The drawing under review shows one solid part. Ordinate dimensions are in mm from its lowest x, y, z. A direction names the side the tool comes from. Round coordinates to 2 decimals unless told otherwise and drop trailing zeros. Order: outer loops, then holes, each group sorted by start corner. A loop starts at its lowest first (then second) coordinate and runs counter-clockwise, first axis right, second up. Notation, with made-up numbers: M 61,80.25 L 85,80.25 A32 cw 85,115.25 Z; hole C -2,-28.5 d2. An arc over 180 degrees is marked long. Use a Markdown table: item, result.
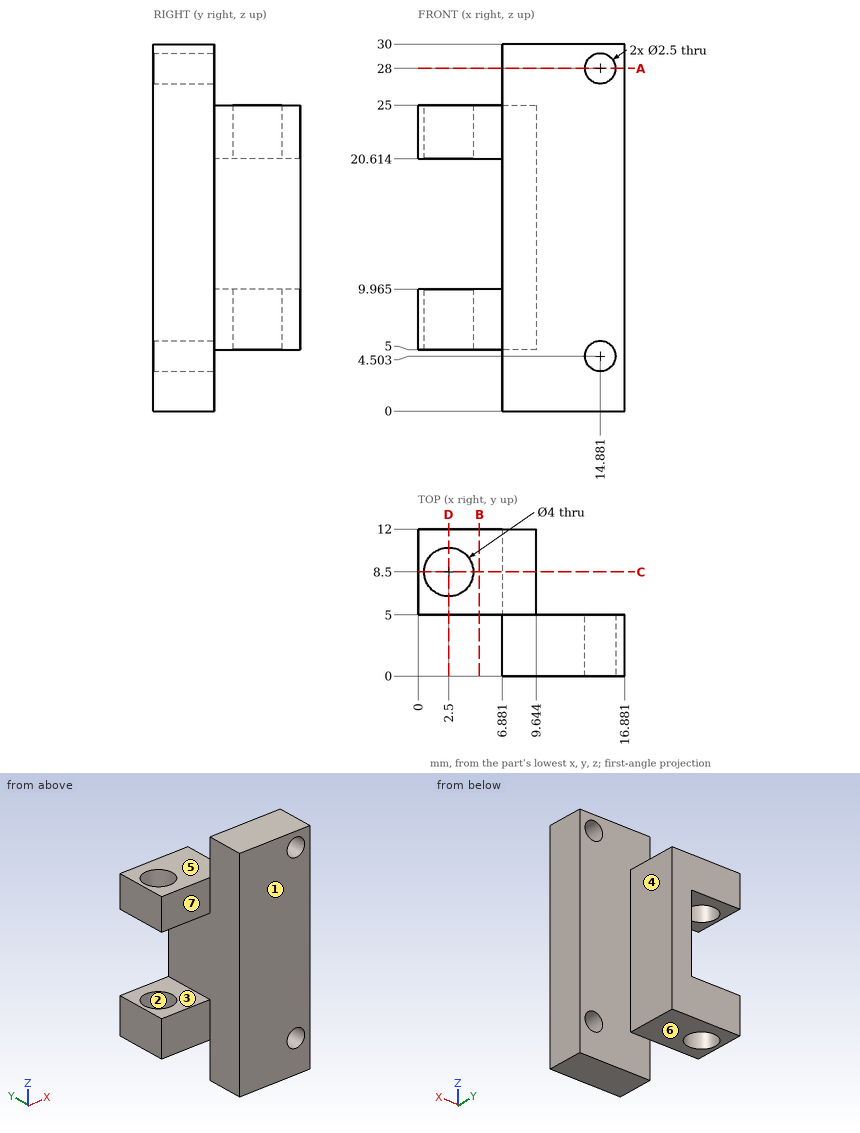
Q1. Machinability: for the marked faces 4, 5, 6 and 7, which of the approach directions +Z, -Z, +X, -X, +Y, -Y give a long, thin tool a straight path to every point of the face, cutting with its end or side? Answer none if there is none.
Determined:
| item | result |
|---|---|
| face 4 | +Z, -Z, +X, +Y |
| face 5 | +Z, +X, -X, +Y |
| face 6 | -Z, +X, -X, +Y |
| face 7 | +Z, -Z, -X, -Y |
Q2. Add section C-C (y = 8.5). Write out the cut boundary in (x, z) (1 decimal).
Determined:
| item | result |
|---|---|
| outline | M 0,5 L 0.5,5 L 0.5,10 L 0,10 Z; M 0,20.6 L 0.5,20.6 L 0.5,25 L 0,25 Z; M 4.5,5 L 9.6,5 L 9.6,25 L 4.5,25 L 4.5,20.6 L 6.9,20.6 L 6.9,10 L 4.5,10 Z |
Q3. Add section D-D (x = 2.5). Write out the cut boundary in (y, z) (1 decimal).
Determined:
| item | result |
|---|---|
| outline | M 5,5 L 6.5,5 L 6.5,10 L 5,10 Z; M 5,20.6 L 6.5,20.6 L 6.5,25 L 5,25 Z; M 10.5,5 L 12,5 L 12,10 L 10.5,10 Z; M 10.5,20.6 L 12,20.6 L 12,25 L 10.5,25 Z |
Q4. Add section B-B (x = 5). Write out the cut boundary in (y, z) (1 decimal).
Determined:
| item | result |
|---|---|
| outline | M 5,5 L 12,5 L 12,10 L 5,10 Z; M 5,20.6 L 12,20.6 L 12,25 L 5,25 Z |
Q5. Clearance check with flat-ended pins moving along their axes: pin 1 (4 mm diameter, centred on x = 2.5, z = 7.5, fed in from -Y); pin 2 (2 mm diameter, centred on x = 5, y = 8.5, fed in from -Z); pin 3 (1.5 mm diameter, centred on x = 14.88, z = 4.5, fed in from -Y); pin 4 (6 mm diameter, centred on x = 9.5, y = 9, fed in from +Z). State where each tip first meets the part, or that it passes through.
Determined:
| item | result |
|---|---|
| pin 1 | stops at y = 5 |
| pin 2 | stops at z = 5 |
| pin 3 | passes through |
| pin 4 | stops at z = 25 |
Q6. Draft analysis for pull direction Y (two halves, no side actions). For the marked faces 1, 2 and 3, state which applies: pulls with the +Y half, pulls with the -Y half, needs draft (parallel to the pull), parting line crosses it, or undercut.
Determined:
| item | result |
|---|---|
| face 1 | pulls with the -Y half |
| face 2 | undercut |
| face 3 | needs draft |
Q7. Wall thickness on line 1 along Z through (x, y) = (15, 1.5) (1 decimal); line 2 along X through (y, z) = (2.35, 28); line 3 along Z through (x, y) = (5.75, 10.25) (1 decimal): over which ranges is each line inside the solid? List them lowest first. Write a range as [from, to].
Determined:
| item | result |
|---|---|
| line 1 | z = [0, 3.3], [5.7, 26.8], [29.2, 30] |
| line 2 | x = [6.88, 13.63], [16.13, 16.88] |
| line 3 | z = [5, 10], [20.6, 25] |
Q8. Add section A-A (z = 28). Write out the cut boundary in (x, y).
Determined:
| item | result |
|---|---|
| outline | M 6.88,0 L 13.63,0 L 13.63,5 L 6.88,5 Z; M 16.13,0 L 16.88,0 L 16.88,5 L 16.13,5 Z |
